Geometry check sheet. Reference: the model listing, model coordinates, mm. A direction names the side the tool comes from. Round coordinates to 2 decimals unless told otherwise and drop trailing zeros. Write each loop counter-clockwise with the first axis right and the second up, starting at its lowest first coordinate (ties: lowest second). Pieces come first, ordered by that corner, then holes. Notation, with made-up numbers: (11.5, 0.5) - (29.5, 0.5) arc R19 cw to (29.5, 36.5) - close; hole circle Ø3 at (78, 45.25). An arc over 180 degrees is marked (long way). One line per question, with ' | ' between items. Start each with the question number.
from build123d import *

# Parameters (mm, degrees)
SKETCH1_R           = 20
BOSS_EXTRUDE1_DEPTH = 50


with BuildPart() as part:
    # Sketch1 → Boss-Extrude1 (new body, symmetric)
    with BuildSketch(Plane.XY):
        Circle(SKETCH1_R)
        with BuildLine():
            Line((2.5, 9.682458366), (2.5, 13))
            Line((2.5, 13), (-2.5, 13))
            Line((-2.5, 13), (-2.5, 9.682458366))
            ThreePointArc((-2.5, 9.682458366), (0, -10), (2.5, 9.682458366))
        make_face(mode=Mode.SUBTRACT)
    extrude(amount=BOSS_EXTRUDE1_DEPTH, both=True)


solid = part.part
Q1. Section check C-C, the plane z = 0. Record the cut outline in (x, y), then the cut area to 3 significant figures.
Q2. Thickness scan on line 1 (Y direction, x = 0, z = -29); line 2 (X direction, y = 4, z = -5.5); line 3 (Y direction, x = 3, z = 42.5). Record the ranges inside material, lowest first.
Q3. Section check D-D, the plane y = -12. Record the cut outline in (x, z), then the cut area to 3 significant figures.
Q4. Draft check along Y on faces 3 (the flat face through (-5, 9, -50)), 4 (the cylindrical face through (-4.336, -19.524, 0.7)), 5 (the flat face through (0, 13, 1)). Enter one of: pulls with the +Y half, pulls with the -Y half, needs draft (parallel to the pull), parting line crosses it, or undercut.
Q5. Section check B-B, the plane x = 0. Record the cut outline in (y, z).
Q6. Go/stop test with flat-tipped pins: P1, Ø1.7, axis at y = 12, z = 19, coming from the +X side; P2, Ø5.5, axis at x = 1, z = -20, coming from the -Y side; P3, Ø3, axis at y = 2, z = -31.5, coming from the -X side. Record where each tip stops, or that it passes through.
Q7. Section check A-A, the plane y = 0. Record the cut outline in (x, z), then the cut area to 3 significant figures.
Q8. Set-up check for faces 1 (the flat face through (-2.5, 11, 1)), 2 (the flat face through (-5, 9, 50)): record each of +Z, -Z, +X, -X, +Y, -Y from which the full face is reachable in a straight line by a thin tool's end or side.
Result sheet:
1) outline: circle Ø40 at (0, 0); hole (-2.5, 9.68) arc R10 ccw (long way) to (2.5, 9.68) - (2.5, 13) - (-2.5, 13) - close | area: 927 mm²
2) line 1: -20 to -10, 13 to 20 | line 2: -19.6 to -9.17, 9.17 to 19.6 | line 3: -19.77 to -9.54, 9.54 to 19.77
3) outline: (-16, -50) - (16, -50) - (16, 50) - (-16, 50) - close | area: 3,200 mm²
4) face 3: needs draft | face 4: parting line crosses it | face 5: undercut
5) outline: (-20, -50) - (-10, -50) - (-10, 50) - (-20, 50) - close; (13, -50) - (20, -50) - (20, 50) - (13, 50) - close
6) P1: x = 16.6 | P2: y = -20 | P3: x = -19.99
7) outline: (-20, -50) - (-10, -50) - (-10, 50) - (-20, 50) - close; (10, -50) - (20, -50) - (20, 50) - (10, 50) - close | area: 2,000 mm²
8) face 1: +Z, -Z | face 2: +Z, +X, -X, +Y, -Y
